```python
from build123d import *

# Parameters (mm, degrees)
SKETCH1_W           = 55
SKETCH1_H           = 106
SKETCH1_W_2         = 24.5
SKETCH1_H_2         = 12
BOSS_EXTRUDE1_DEPTH = 4.5
SKETCH2_R           = 1.6
CUT_EXTRUDE1_DEPTH  = 60.879044749
SKETCH3_W           = 10.5
SKETCH3_H           = 4.7
CUT_EXTRUDE2_DEPTH  = 60.879044749


with BuildPart() as part:
    # Sketch1 → Boss-Extrude1 (new body)
    with BuildSketch(Plane.XY):
        Rectangle(SKETCH1_W, SKETCH1_H)
        with Locations((-13.5, 22.5)):
            Rectangle(SKETCH1_W_2, SKETCH1_H_2, mode=Mode.SUBTRACT)
        with Locations((13.5, 22.5)):
            Rectangle(SKETCH1_W_2, SKETCH1_H_2, mode=Mode.SUBTRACT)
        with Locations((13.5, -22.5)):
            Rectangle(SKETCH1_W_2, SKETCH1_H_2, mode=Mode.SUBTRACT)
        with Locations((-13.5, -22.5)):
            Rectangle(SKETCH1_W_2, SKETCH1_H_2, mode=Mode.SUBTRACT)
    extrude(amount=BOSS_EXTRUDE1_DEPTH)

    # Sketch2 → Cut-Extrude1 (cut, through all)
    with BuildSketch(Plane.XY.offset(4.5)):
        with Locations((-15, 33)):
            Circle(SKETCH2_R)
        with Locations(Location((15, 33, 0), (0, 0, 180))):
            Circle(SKETCH2_R)
        with Locations((15, -33)):
            Circle(SKETCH2_R)
        with Locations(Location((-15, -33, 0), (0, 0, 180))):
            Circle(SKETCH2_R)
    extrude(amount=-CUT_EXTRUDE1_DEPTH, mode=Mode.SUBTRACT)

    # Sketch3 → Cut-Extrude2 (cut, through all)
    with BuildSketch(Plane.XY.offset(4.5)):
        with Locations((-14, 0)):
            Rectangle(SKETCH3_W, SKETCH3_H)
        with Locations((14, 0)):
            Rectangle(SKETCH3_W, SKETCH3_H)
    extrude(amount=-CUT_EXTRUDE2_DEPTH, mode=Mode.SUBTRACT)


solid = part.part
```
The model under review builds one solid part; all positions refer to its coordinate system, in mm. A direction names the side the tool comes from. Round coordinates to 2 decimals unless told otherwise and drop trailing zeros. Loops run counter-clockwise (first coordinate to the right, second up) from the corner with the lowest first, then second, coordinate; pieces in that order, holes last. Notation, with made-up numbers: (-0.75, 84.25) -> (20.25, 84.25) arc R19 cw to (20.25, 98.25) -> close; hole circle Ø9 at (83, 48). An arc over 180 degrees is marked (long way). Answer as a JSON object with one key per item and string values. Group by question number.
1) For line 1 (Y direction, x = -7, z = 2.4); line 2 (Y direction, x = 15, z = 2.45); line 3 (X direction, y = -0.5, z = 1.1), list the stretches that pass through material, from the lowest coordinate up. Write a range as [from, to].
2) For faces 1 (the face through (-25.75, 22, 2)), 2 (the face through (0, 1, 4.5)), list the 3-axis set-ups (+Z, -Z, +X, -X, +Y, -Y) from which the entire face can be reached by the end or side of a thin tool; tool diameter is ignored.
3) We need section B-B on x = -12. Write out the cut boundary in (y, z), then the cut area to 3 significant figures.
4) We need section A-A on x = 22. Write out the cut boundary in (y, z), then the cut area to 3 significant figures.
5) We need section C-C on z = 2.1. Give the number of separate pieces and of enclosed holes in the cut face, then the cut area to 3 significant figures.
6) We need section D-D on y = 33. Write out the cut boundary in (x, z).
7) Mouldability with a two-part tool opening along X and no side actions: class faces 3 (the face through (27.5, -1, 2)), 4 (the face through (0, -53, 2)), 5 (the face through (14, -2.35, 2)) as released by +X, released by -X, zero draft, split by the parting line, or undercut.
Result set:
{
 "1": {"line 1": "[-53, -28.5], [-16.5, 16.5], [28.5, 53]", "line 2": "[-53, -34.6], [-31.4, -28.5], [-16.5, -2.35], [2.35, 16.5], [28.5, 31.4], [34.6, 53]", "line 3": "[-27.5, -19.25], [-8.75, 8.75], [19.25, 27.5]"},
 "2": {"face 1": "+Z, -Z", "face 2": "+Z, +X, -X, +Y, -Y"},
 "3": {"outline": "(-53, 0) -> (-28.5, 0) -> (-28.5, 4.5) -> (-53, 4.5) -> close; (-16.5, 0) -> (-2.35, 0) -> (-2.35, 4.5) -> (-16.5, 4.5) -> close; (2.35, 0) -> (16.5, 0) -> (16.5, 4.5) -> (2.35, 4.5) -> close; (28.5, 0) -> (53, 0) -> (53, 4.5) -> (28.5, 4.5) -> close", "area": "348 mm²"},
 "4": {"outline": "(-53, 0) -> (-28.5, 0) -> (-28.5, 4.5) -> (-53, 4.5) -> close; (-16.5, 0) -> (16.5, 0) -> (16.5, 4.5) -> (-16.5, 4.5) -> close; (28.5, 0) -> (53, 0) -> (53, 4.5) -> (28.5, 4.5) -> close", "area": "369 mm²"},
 "5": {"separate pieces": "1", "enclosed holes": "10", "area": "4,520 mm²"},
 "6": {"outline": "(-27.5, 0) -> (-16.6, 0) -> (-16.6, 4.5) -> (-27.5, 4.5) -> close; (-13.4, 0) -> (13.4, 0) -> (13.4, 4.5) -> (-13.4, 4.5) -> close; (16.6, 0) -> (27.5, 0) -> (27.5, 4.5) -> (16.6, 4.5) -> close"},
 "7": {"face 3": "released by +X", "face 4": "zero draft", "face 5": "undercut"}
}
